Work out the finished part from the listing and answer in its coordinate system (mm). Face numbers are marked on the shaded views. A direction names the side the tool comes from. Coordinates: 2 decimals unless noted, no trailing zeros. Write each loop counter-clockwise with the first axis right and the second up, starting at its lowest first coordinate (ties: lowest second). Pieces come first, ordered by that corner, then holes. Notation, with made-up numbers: M -38.75,31.25 L -2.75,31.25 A18 cw -2.75,60.25 Z; hole C -1,37 d7. An arc over 180 degrees is marked long. Use CSV: the item, a comma, the result in double quotes.
Autodesk Inventor part; units mm, degrees
ref_plane "YZ Plane" through (0, 0, 0) normal (1, 0, 0) x (0, 1, 0)
ref_plane "XZ Plane" through (0, 0, 0) normal (0, 1, 0) x (-1, 0, 0)
ref_plane "XY Plane" through (0, 0, 0) normal (0, 0, 1) x (1, 0, 0)
sketch "Sketch1" plane through (0, 0, 0) normal (0, 0, 1) x (1, 0, 0)
  line L0 (0, 0) -> (25.4, 0)
  line L1 (25.4, 0) -> (25.4, 25.4)
  line L2 (25.4, 25.4) -> (0, 25.4)
  line L3 (0, 25.4) -> (0, 0)
  line L4 (3.175, 3.175) -> (22.225, 3.175)
  line L5 (22.225, 3.175) -> (22.225, 22.225)
  line L6 (22.225, 22.225) -> (3.175, 22.225)
  line L7 (3.175, 22.225) -> (3.175, 3.175)
  dimension "d0" = 25.4
  dimension "d1" = 25.4
  dimension "d2" = 3.175
  dimension "d3" = 3.175
  dimension "d4" = 3.175
  dimension "d5" = 3.175
extrude "Extrusion1" add sketch "Sketch1" along normal blind 152.4
sketch "Sketch2" plane through (25.4, 0, 0) normal (1, 0, 0) x (0, 0, -1)
  line L0 (-152.4, 25.4) -> (-152.4, 0)
  line L1 (0, 0) -> (-152.4, 0)
  line L2 (0, 0) -> (0, 25.4)
  line L3 (0, 25.4) -> (-152.4, 25.4)
  circle A0 centre (-12.7, 12.7) radius 4.7625
  arc A1 (-12.7, 0) -> (-12.7, 25.4) centre (-12.7, 12.7) ccw
  dimension "d8" = 9.525
  dimension "d9" = 12.7
  dimension "d10" = 12.7
extrude "Extrusion2" cut sketch "Sketch2" against normal blind 25.4 contours L3 L2 A1 | A1 L2 L1 | A0
equation "\"d2\" = d5"
equation "\"d3\" = d2"
equation "\"d5\" = d4"
equation "\"d10\" = d9"
properties part number "8 ball top arm tube"
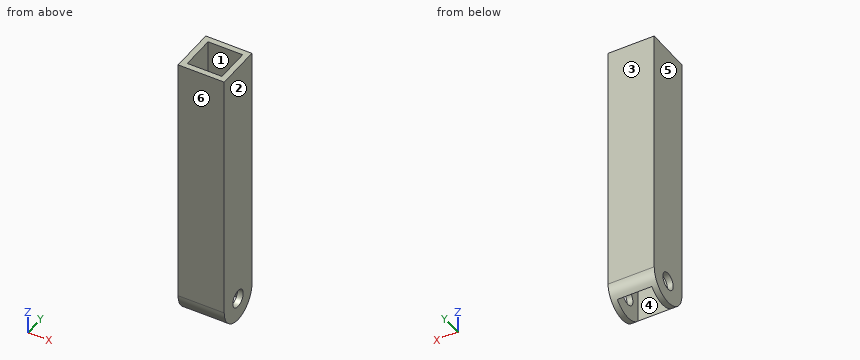
Item 1: Given pin 1 (6 mm diameter, centred on x = 13, y = 8.5, fed in from -Z); pin 2 (3 mm diameter, centred on x = 4, y = 6.5, fed in from -Z), each flat-ended and moving along its own axis, determine where each tip first touches the part or whether it passes through.
Answer:
pin 1,"passes through"
pin 2,"stops at z = 1"
Item 2: The part is cut by section B-B (y = 12.7). Write down the section's boundary in (x, z) (1 decimal), then the cut area to 3 significant figures.
Answer:
outline,"M 0,0 L 3.2,0 L 3.2,7.9 L 0,7.9 Z; M 0,17.5 L 3.2,17.5 L 3.2,152.4 L 0,152.4 Z; M 22.2,0 L 25.4,0 L 25.4,7.9 L 22.2,7.9 Z; M 22.2,17.5 L 25.4,17.5 L 25.4,152.4 L 22.2,152.4 Z"
area,"907 mm2"
Item 3: For a pull along Y with two mould halves and no side action, classify the marked faces 3, 4, 5 and 6 as released by +Y, released by -Y, zero draft, split by the parting line, or undercut.
Answer:
face 3,"released by +Y"
face 4,"undercut"
face 5,"zero draft"
face 6,"released by -Y"
Item 4: The part is cut by section C-C (z = 61). Write down the section's boundary in (x, y) (3 decimals).
Answer:
outline,"M 0,0 L 25.4,0 L 25.4,25.4 L 0,25.4 Z; hole M 3.175,3.175 L 22.225,3.175 L 22.225,22.225 L 3.175,22.225 Z"
Item 5: The part is cut by section A-A (x = 10). Write down the section's boundary in (y, z) (3 decimals).
Answer:
outline,"M 0,12.7 A12.7 ccw 3.175,4.3 L 3.175,152.4 L 0,152.4 Z; M 22.225,4.3 A12.7 ccw 25.4,12.7 L 25.4,152.4 L 22.225,152.4 Z"
Item 6: Consider probe 1 along X at (y, z) = (6.5, 9) (3 decimals); probe 2 along Y at (x, z) = (1.2, 12.7). Determine where each line is inside the solid, lowest interval first.
Answer:
probe 1,"x = 0 to 3.175, 22.225 to 25.4"
probe 2,"y = 0 to 7.94, 17.46 to 25.4"
Item 7: A tool of negligible diameter and unlimited length cuts with its end or side. For the marked faces 1 and 2, from which of +Z, -Z, +X, -X, +Y, -Y can it reach the whole face along a straight path? Write none if from no direction.
Answer:
face 1,"+Z, -Z"
face 2,"+Z, -Z, +X, +Y, -Y"
Item 8: The part is cut by section D-D (y = 20). Write down the section's boundary in (x, z) (3 decimals).
Answer:
outline,"M 0,2.308 L 3.175,2.308 L 3.175,152.4 L 0,152.4 Z; M 22.225,2.308 L 25.4,2.308 L 25.4,152.4 L 22.225,152.4 Z"
